Check sheet for the modelled part. Datum: model origin and axes. Units: mm. Coordinates: 2 decimals unless noted, no trailing zeros.
1. Draft check along X on faces 1 (the flat face through (-25, -1, 3)), 2 (the flat face through (0.35, -1, 2)), 3 (the flat face through (0, -2, 4)). Enter one of: released by +X, released by -X, zero draft, split by the parting line, or undercut.
2. Gauge pin test, flat ends, axial feed: pin 1 Ø2 at (x, z) = (-13.5, 3) entering from +Y; pin 2 Ø0.6 at (x, y) = (-12, -1) entering from +Z; pin 3 Ø1 at (x, y) = (-20.5, -0.5) entering from -Z. Record the tip position at first contact, or that the pin passes through.
3. Thickness scan on line 1 (X direction, y = -0.55, z = 2.35); line 2 (Y direction, x = -21, z = 2.85); line 3 (Z direction, x = -21, y = -0.4). Record the ranges inside material, lowest first.
```python
from build123d import *

# Parameters (mm, degrees)
F1_DEPTH = 2
F2_W     = 0.01
F2_H     = 2
F3_DEPTH = 0.01
F4_W     = 0.01
F4_H     = 2
F5_DEPTH = 0.01


with BuildPart() as f1:
    # F0 (on Front) → F1 (new body)
    with BuildSketch(Plane.XZ):
        Polygon((0.35, 3), (0.35, 0), (25, 0), (25, 5), (0, 5), (-25, 5), (-25, 0), (-0.35, 0), (-0.35, 3), (0, 3), align=None)
    extrude(amount=F1_DEPTH)

    # F2 (on face) → F3 (join)
    with BuildSketch(Plane(origin=(0, 0, 0), x_dir=(1, 0, 0), z_dir=(0, 0, -1))):
        with Locations((16.446504, 0.998741)):
            Rectangle(F2_W, F2_H)
        with Locations((-16.628518, 1)):
            Rectangle(F2_W, F2_H)
    extrude(amount=F3_DEPTH)

    # F4 (on face) → F5 (join)
    with BuildSketch(Plane.XY.offset(5)):
        with Locations((0, -1)):
            Rectangle(F4_W, F4_H)
    extrude(amount=F5_DEPTH)


solid = f1.part
```
Data:
1. face 1: released by -X
1. face 2: undercut
1. face 3: zero draft
2. pin 1: stops at y = 0
2. pin 2: stops at z = 5
2. pin 3: stops at z = 0
3. line 1: x = -25 to -0.35, 0.35 to 25
3. line 2: y = -2 to 0
3. line 3: z = 0 to 5
